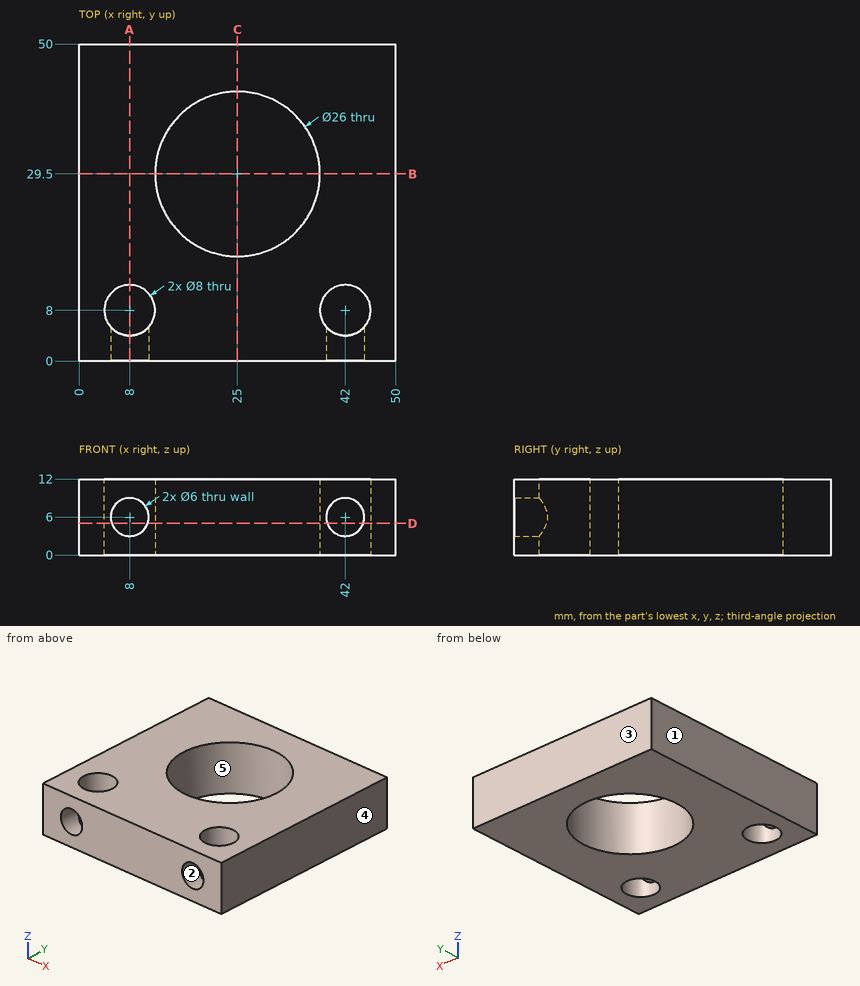
Verification items for this drawing (mm, ordinates from the low corner). A direction names the side the tool comes from. Coordinates: 2 decimals unless noted, no trailing zeros. Write each loop counter-clockwise with the first axis right and the second up, starting at its lowest first coordinate (ties: lowest second). Pieces come first, ordered by that corner, then holes. Notation, with made-up numbers: M 23.25,65 L 29.25,65 A17 cw 29.25,74 Z; hole C -27.75,-9 d7. An arc over 180 degrees is marked long. Use CSV: the item, a comma, the result in double quotes.
Q1. Set-up check for the marked faces 1 and 2: record each of +Z, -Z, +X, -X, +Y, -Y from which the full face is reachable in a straight line by a thin tool's end or side.
Computed values:
face 1,"+Z, -Z, -X, +Y, -Y"
face 2,"-Y"
Q2. Section check B-B, the plane y = 29.5. Enter the section's corners in (x, z), and give its area (3 significant figures).
Computed values:
outline,"M 0,0 L 12,0 L 12,12 L 0,12 Z; M 38,0 L 50,0 L 50,12 L 38,12 Z"
area,"288 mm²"
Q3. Mould release check, pull along X, two halves, no side actions. Record for the marked faces 3, 4 and 5: pulls with the +X half, pulls with the -X half, needs draft (parallel to the pull), parting line crosses it, or undercut.
Computed values:
face 3,"needs draft"
face 4,"pulls with the +X half"
face 5,"undercut"
Q4. Section check D-D, the plane z = 5. Enter the section's corners in (x, y).
Computed values:
outline,"M 0,0 L 5.17,0 L 5.17,5.17 A4 cw long 10.83,5.17 L 10.83,0 L 39.17,0 L 39.17,5.17 A4 cw long 44.83,5.17 L 44.83,0 L 50,0 L 50,50 L 0,50 Z; hole C 25,29.5 d26"
Q5. Section check A-A, the plane x = 8. Enter the section's corners in (y, z).
Computed values:
outline,"M 0,0 L 4,0 L 4,3 L 0,3 Z; M 0,9 L 4,9 L 4,12 L 0,12 Z; M 12,0 L 50,0 L 50,12 L 12,12 Z"
Q6. Section check C-C, the plane x = 25. Enter the section's corners in (y, z).
Computed values:
outline,"M 0,0 L 16.5,0 L 16.5,12 L 0,12 Z; M 42.5,0 L 50,0 L 50,12 L 42.5,12 Z"
Q7. Go/stop test with a flat-tipped pin: P1, Ø5.5, axis at x = 8, z = 6, coming from the -Y side. Record where the tip stops, or that it passes through.
Computed values:
P1,"y = 10.9"
Q8. Thickness scan on line 1 along X through (y, z) = (3.5, 6.25); line 2 along Y through (x, z) = (25, 3.5); line 3 along Z through (x, y) = (8, 3.7). Record the ranges inside material, lowest first. Write a range as [from, to].
Computed values:
line 1,"[0, 5.01], [10.99, 39.01], [44.99, 50]"
line 2,"[0, 16.5], [42.5, 50]"
line 3,"[0, 3], [9, 12]"
